Here's how the part is built. I have some questions about the finished solid (model axes, mm). Face numbers are marked on the shaded views. A direction names the side the tool comes from. Round coordinates to 2 decimals unless told otherwise and drop trailing zeros. Write each loop counter-clockwise with the first axis right and the second up, starting at its lowest first coordinate (ties: lowest second). Pieces come first, ordered by that corner, then holes. Notation, with made-up numbers: (65, 31.25) -> (103, 31.25) arc R29 ccw to (103, 53.25) -> close; hole circle Ø7 at (26.25, 75.5). An arc over 180 degrees is marked (long way). Answer in a Markdown table with one row per item.
from build123d import *

# Parameters (mm, degrees)
CHANFREIN1_SIZE = 1


with BuildPart() as part:
    # Esquisse1 → Révolution2 (revolve)
    with BuildSketch(Plane.XY, mode=Mode.PRIVATE) as r_volution2_sk:
        Polygon((438.964577225, -15), (438.964577225, -12), (441.464577225, -12), (441.464577225, -15), (451.464577225, -15), (451.464577225, -10), (450.464577225, -10), (450.464577225, 0), (316.5, 0), (316.5, -7.6), (313.5, -7.6), (313.5, -9.6), (399.5, -9.6), (399.5, -15), (410, -15), (410, -29), (415.5, -19.5), (419.5, -19.5), (419.5, -18.5), (423.5, -18.5), (421.464577225, -15), align=None)
    revolve(r_volution2_sk.sketch.rotate(Axis((313.5, 0, 0), (-1, 0, 0)), 270), axis=Axis((313.5, 0, 0), (-1, 0, 0)))

    # Chanfrein1
    chanfrein1_edges = [part.edges().sort_by_distance(p)[0] for p in [
        (438.964577225, 0, 15),
        (441.464577225, 0, 15),
        (451.464577225, 0, 15),
        (451.464577225, 0, 10),
    ]]
    chamfer(chanfrein1_edges, length=CHANFREIN1_SIZE - 0.0001)  # a hair under: the kernel refuses the full size


solid = part.part
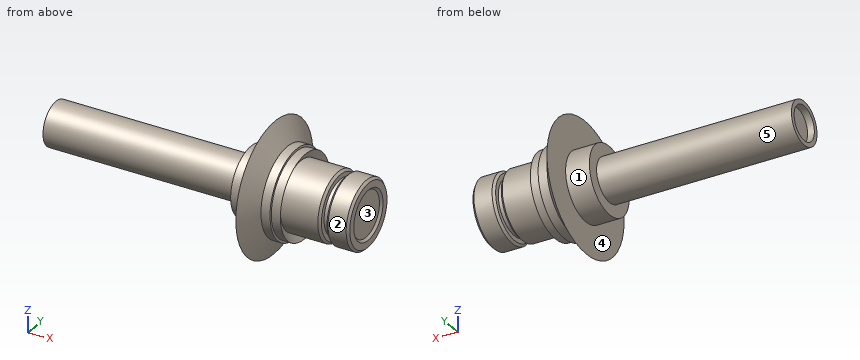
1) I want a section at A-A, the plane x = 377. List the corners of the cut face in (y, z) for me.
Response:
| item | result |
|---|---|
| outline | circle Ø19.2 at (0, 0) |
2) For pin 1 (3 mm diameter, centred on y = 3.5, z = 21, fed in from -X); pin 2 (2 mm diameter, centred on x = 425, z = 13, fed in from +Y); pin 3 (10 mm diameter, centred on x = 392, y = 1, fed in from +Z), each with a flat end and sliding along its axis, tell me the tip position at first contact or that it passes through.
Response:
| item | result |
|---|---|
| pin 1 | stops at x = 410 |
| pin 2 | stops at y = 9 |
| pin 3 | stops at z = 9.6 |
3) We'd pull the mould along Z, two halves only. Please class the marked faces 3, 4 and 5: +Z half, -Z half, draft (parallel to the pull), parting line (faces both ways), or undercut.
Response:
| item | result |
|---|---|
| face 3 | undercut |
| face 4 | draft |
| face 5 | parting line |
4) I need wall thicknesses on line 1 (Y direction, x = 314, z = 0); line 2 (Y direction, x = 450, z = 0); line 3 (X direction, y = 5, z = 2.5). Which ranges of each line are inside material? Lowest first, please. Write a range as [from, to].
Response:
| item | result |
|---|---|
| line 1 | y = [-9.6, -7.6], [7.6, 9.6] |
| line 2 | y = [-15, 15] |
| line 3 | x = [316.5, 450.46] |
5) Which directions (+Z, -Z, +X, -X, +Y, -Y) give clear straight access to the entire face, cutting with the end or side of a thin tool? Please do the marked faces 1 and 2.
Response:
| item | result |
|---|---|
| face 1 | -X |
| face 2 | +X |
